from build123d import *

# Parameters (mm, degrees)
F1_DEPTH = 0.9652
F2_W     = 1.905
F2_H     = 15.0368
F3_DEPTH = 2.9718
F2_R     = 1.0033
F2_R_2   = 0.8037883442
F4_DEPTH = 1.9558
F5_W     = 1.8288
F5_H     = 15.0368
F6_DEPTH = 0.381
F7_R     = 0.254


with BuildPart() as f1:
    # F0 (on Top) → F1 (new body)
    with BuildSketch(Plane.XY):
        Polygon((-2.7559, -7.5184), (2.7559, -7.5184), (2.7559, 7.5184), (0.8509, 7.5184), (-2.7559, 7.5184), (-2.7559, 1.905), (-23.0759, 1.905), (-21.0439, -2.035223273), (-2.7559, -2.035223273), align=None)
    extrude(amount=F1_DEPTH)

    # F2 (on face) → F3 (join)
    with BuildSketch(Plane.XY.offset(0.9652)):
        with Locations((1.8034, 0)):
            Rectangle(F2_W, F2_H)
    extrude(amount=F3_DEPTH)

    # F2 (on face) → F4 (join)
    with BuildSketch(Plane.XY.offset(0.9652)):
        with Locations((-10.0076, 0)):
            Circle(F2_R)
        with Locations((-10.0076, 0)):
            Circle(F2_R_2, mode=Mode.SUBTRACT)
    extrude(amount=F4_DEPTH)

    # F5 (on face) → F6 (cut)
    with BuildSketch(Plane(origin=(0, 0, 0), x_dir=(1, 0, 0), z_dir=(0, 0, -1))):
        with Locations((0.0654817199, 0)):
            Rectangle(F5_W, F5_H)
    extrude(amount=-F6_DEPTH, mode=Mode.SUBTRACT)

    # F7
    f7_edges = [f1.edges().sort_by_distance(p)[0] for p in [
        (-23.0759, 1.905, 0.4826),
        (-21.0439, -2.035223, 0.4826),
        (-2.7559, -7.5184, 0.4826),
        (-2.7559, 7.5184, 0.4826),
        (-2.7559, -2.035223, 0.4826),
        (-2.7559, 1.905, 0.4826),
        (-1.802409, 7.5184, 0),
        (1.867891, 7.5184, 0),
        (2.7559, 0, 0),
        (-2.7559, 4.7117, 0),
        (-2.7559, -4.776812, 0),
        (-1.802409, -7.5184, 0),
        (1.867891, -7.5184, 0),
        (-11.8999, -2.035223, 0),
        (-12.9159, 1.905, 0),
    ]]
    fillet(f7_edges, radius=F7_R)


solid = f1.part
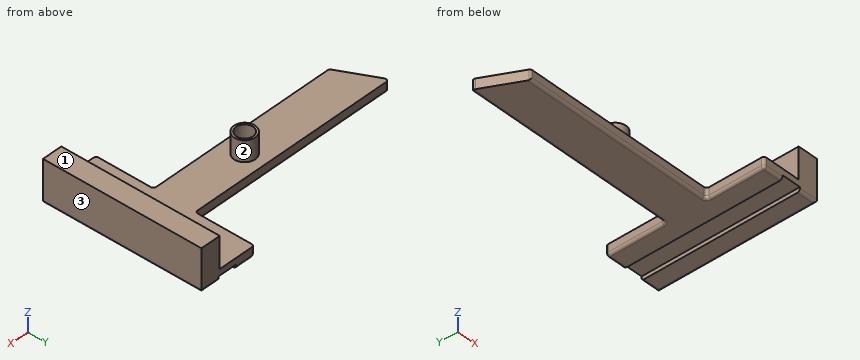
Part model, mm, in its own coordinate system. Face numbers are marked on the shaded views. Coordinates: 2 decimals unless noted, no trailing zeros. Loops run counter-clockwise (first coordinate to the right, second up) from the corner with the lowest first, then second, coordinate; pieces in that order, holes last. Notation, with made-up numbers: (6.25, 77) - (10.25, 77) arc R28 cw to (10.25, 116) - close; hole circle Ø7 at (-29.75, 45.5). An arc over 180 degrees is marked (long way). Write each question's results on one line, items separated by ' | '. Start each with the question number.
Q1. Slice it at B-B on y = -5.5. Give the cut face in (x, z).
Q2. Slice it at C-C on x = -4.5. Give the cut face in (y, z) (3 decimals), and give its area (3 significant figures).
Q3. Slice it at D-D on y = 0. Give the cut face in (x, z), and give its area (3 significant figures).
Q4. Two-plate mould, pull along X, no slides. Class the marked faces 1, 2 and 3: +X half, -X half, draft (parallel to the pull), parting line (faces both ways), or undercut.
Q5. Probe line 1 along X through (y, z) = (0.25, 1.6); line 2 along Y through (x, z) = (-15.75, 0.65) (3 decimals); line 3 along Z through (x, y) = (-7.75, 0.75). List the from-to ranges inside material, lowest first.
Q6. Drop flat-ended pins along their axis: pin 1 Ø5 at (x, y) = (-12.5, 1.5) entering from +Z; pin 2 Ø0.8 at (y, z) = (-5, 0.5) entering from -X; pin 3 Ø4 at (x, y) = (-12, 2.5) entering from +Z; pin 4 Ø4 at (x, y) = (-18, 4) entering from -Z. Give the stop position or say it passes through.
Q7. Slice it at A-A on z = 2.6. Give the cut face in (x, y).
Answer:
1) outline: (-2.76, 0.25) arc R0.25 ccw to (-2.5, 0) - (-0.85, 0) - (-0.85, 0.38) - (0.98, 0.38) - (0.98, 0) - (2.5, 0) arc R0.25 ccw to (2.76, 0.25) - (2.76, 3.94) - (0.85, 3.94) - (0.85, 0.97) - (-2.76, 0.97) - close
2) outline: (-2.035, 0.254) arc R0.254 ccw to (-1.781, 0) - (1.651, 0) arc R0.254 ccw to (1.905, 0.254) - (1.905, 0.965) - (-2.035, 0.965) - close | area: 3.78 mm2
3) outline: (-22.09, 0) - (-0.85, 0) - (-0.85, 0.38) - (0.98, 0.38) - (0.98, 0) - (2.5, 0) arc R0.25 ccw to (2.76, 0.25) - (2.76, 3.94) - (0.85, 3.94) - (0.85, 0.97) - (-9, 0.97) - (-9, 2.92) - (-9.2, 2.92) - (-9.2, 0.97) - (-10.81, 0.97) - (-10.81, 2.92) - (-11.01, 2.92) - (-11.01, 0.97) - (-22.09, 0.97) - close | area: 29.7 mm2
4) face 1: draft | face 2: undercut | face 3: +X half
5) line 1: x = -10.98 to -10.77, -9.24 to -9.04, 0.85 to 2.76 | line 2: y = -2.035 to 1.905 | line 3: z = 0 to 0.97
6) pin 1: stops at z = 2.92 | pin 2: stops at x = -2.76 | pin 3: stops at z = 0.97 | pin 4: passes through
7) outline: circle Ø2.01 at (-10.01, 0); (0.85, -7.52) - (2.76, -7.52) - (2.76, 7.52) - (0.85, 7.52) - close; hole circle Ø1.61 at (-10.01, 0)
